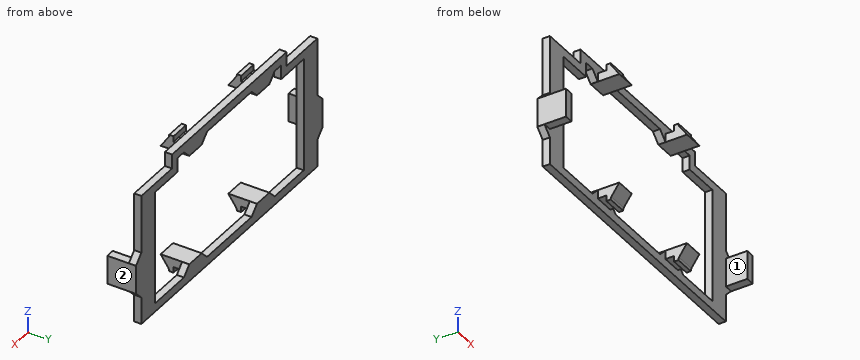
from build123d import *

# Parameters (mm, degrees)
PAD_DEPTH         = 1
SKETCH001_W       = 2.75
SKETCH001_H       = 1.2
PAD001_DEPTH      = 3
PAD001_DEPTH_BACK = 1
CHAMFER_SIZE      = 1.19
SKETCH002_W       = 2.75
SKETCH002_H       = 2
PAD002_DEPTH      = 0.6
FILLET_R          = 0.79
CHAMFER001_SIZE   = 1.19
SKETCH003_W       = 1.2
SKETCH003_H       = 4
PAD003_DEPTH      = 3
PAD003_DEPTH_BACK = 1
CHAMFER002_SIZE   = 1.19


with BuildPart() as part:
    # Sketch → Pad (new body)
    with BuildSketch(Plane.XZ):
        Polygon((-19.5, -9.15), (19.5, -9.15), (19.5, 9.15), (12.7, 9.15), (12.7, 11.15), (-12.7, 11.15), (-12.7, 9.15), (-19.5, 9.15), align=None)
        Polygon((-16.5, -7.95), (16.5, -7.95), (16.5, 7.95), (11.5, 7.95), (11.5, 9.95), (-11.5, 9.95), (-11.5, 7.95), (-16.5, 7.95), align=None, mode=Mode.SUBTRACT)
    extrude(amount=-PAD_DEPTH)

    # Sketch001 → Pad001 (join, two sides)
    with BuildSketch(Plane.XZ) as pad001_sk:
        with Locations((-7.5, 9.35)):
            Rectangle(SKETCH001_W, SKETCH001_H)
        with Locations((7.5, 9.35)):
            Rectangle(SKETCH001_W, SKETCH001_H)
        with Locations((-7.5, -7.35)):
            Rectangle(SKETCH001_W, SKETCH001_H)
        with Locations((7.5, -7.35)):
            Rectangle(SKETCH001_W, SKETCH001_H)
    extrude(amount=PAD001_DEPTH)
    extrude(pad001_sk.sketch, amount=-PAD001_DEPTH_BACK)

    # Chamfer
    chamfer_edges = [part.edges().sort_by_distance(p)[0] for p in [
        (-6.125, 0.5, -7.95),
        (-8.875, 0.5, -7.95),
        (6.125, 0.5, -7.95),
        (8.875, 0.5, -7.95),
        (8.875, 0.5, 9.95),
        (6.125, 0.5, 9.95),
        (-6.125, 0.5, 9.95),
        (-8.875, 0.5, 9.95),
    ]]
    chamfer(chamfer_edges, length=CHAMFER_SIZE)

    # Sketch002 (on DatumPlane) → Pad002 (join)
    with BuildSketch(Plane.XZ.offset(1.2)):
        with Locations((-7.5, 9.75)):
            Rectangle(SKETCH002_W, SKETCH002_H)
        with Locations((7.5, 9.75)):
            Rectangle(SKETCH002_W, SKETCH002_H)
        with Locations((7.5, -7.75)):
            Rectangle(SKETCH002_W, SKETCH002_H)
        with Locations((-7.5, -7.75)):
            Rectangle(SKETCH002_W, SKETCH002_H)
    extrude(amount=PAD002_DEPTH)

    # Fillet
    fillet_edges = [part.edges().sort_by_distance(p)[0] for p in [
        (7.5, -1.8, 9.95),
        (-7.5, -1.8, 9.95),
        (-7.5, -1.8, -7.95),
        (7.5, -1.8, -7.95),
    ]]
    fillet(fillet_edges, radius=FILLET_R)

    # Chamfer001
    chamfer001_edges = [part.edges().sort_by_distance(p)[0] for p in [
        (7.5, -3, 9.95),
        (-7.5, -3, 9.95),
        (-7.5, -3, -7.95),
        (7.5, -3, -7.95),
    ]]
    chamfer(chamfer001_edges, length=CHAMFER001_SIZE)

    # Sketch003 → Pad003 (join, two sides)
    with BuildSketch(Plane.XZ) as pad003_sk:
        with Locations((20.1, -2.15)):
            Rectangle(SKETCH003_W, SKETCH003_H)
        with Locations((-20.1, -2.15)):
            Rectangle(SKETCH003_W, SKETCH003_H)
    extrude(amount=PAD003_DEPTH)
    extrude(pad003_sk.sketch, amount=-PAD003_DEPTH_BACK)

    # Chamfer002
    chamfer002_edges = [part.edges().sort_by_distance(p)[0] for p in [
        (-19.5, 0.5, -4.15),
        (-19.5, 0.5, -0.15),
        (19.5, 0.5, -4.15),
        (19.5, 0.5, -0.15),
    ]]
    chamfer(chamfer002_edges, length=CHAMFER002_SIZE)


solid = part.part
Can you work these out from the model? Positions are in its coordinate system, mm. Face numbers are marked on the shaded views. A direction names the side the tool comes from. Coordinates: 2 decimals unless noted, no trailing zeros. Write each loop counter-clockwise with the first axis right and the second up, starting at its lowest first coordinate (ties: lowest second). Pieces come first, ordered by that corner, then holes. Notation, with made-up numbers: (62, 26.25) - (81, 26.25) arc R17 cw to (81, 58.25) - close; hole circle Ø6 at (18, -22.75). An arc over 180 degrees is marked (long way). Return JSON: item names as keys, results as strings. Group by question number.
Item 1: Which directions (+Z, -Z, +X, -X, +Y, -Y) give clear straight access to the entire face, cutting with the end or side of a thin tool? Please do the marked faces 1 and 2.
Item 2: If we section it at A-A (z = 1.5): Write out the boundary of the cut face in (x, y).
Item 3: Please list where these lines run through material, in increasing order: probe 1 along X at (y, z) = (0.3, 8); probe 2 along X at (y, z) = (-0.25, -2.75); probe 3 along Z at (x, y) = (13.5, 0.2).
Item 4: If we section it at B-B (x = -12): Write out the boundary of the cut face in (y, z), then the cut area to 3 significant figures.
Item 5: If we section it at C-C (y = -0.45): Write out the boundary of the cut face in (x, z) (3 decimals), then the cut area to 3 significant figures.
Item 6: I'm going to push flat-ended pins straight in: pin 1 Ø0.5 at (x, y) = (17, 0.5) entering from +Z; pin 2 Ø2 at (y, z) = (-2, -7.5) entering from -X (3 decimals); pin 3 Ø0.8 at (y, z) = (0.5, 8.5) entering from -X. Where does each tip first touch, or does it pass through?
Item 7: If we section it at D-D (x = -18): Write out the boundary of the cut face in (y, z).
Return value:
{
 "1": {"face 1": "+Z, -Z, -Y", "face 2": "+Z, -Z, +X, +Y, -Y"},
 "2": {"outline": "(-19.5, 0) - (-16.5, 0) - (-16.5, 1) - (-19.5, 1) - close; (16.5, 0) - (19.5, 0) - (19.5, 1) - (16.5, 1) - close"},
 "3": {"probe 1": "x = -19.5 to -11.5, 11.5 to 19.5", "probe 2": "x = -20.7 to -19.5, 19.5 to 20.7", "probe 3": "z = -9.15 to -7.95, 7.95 to 9.15"},
 "4": {"outline": "(0, -9.15) - (1, -9.15) - (1, -7.95) - (0, -7.95) - close; (0, 7.95) - (1, 7.95) - (1, 11.15) - (0, 11.15) - close", "area": "4.40 mm^2"},
 "5": {"outline": "(-20.7, -4.15) - (-19.5, -4.15) - (-19.5, -0.15) - (-20.7, -0.15) - close; (-8.875, -7.95) - (-6.125, -7.95) - (-6.125, -6.75) - (-8.875, -6.75) - close; (-8.875, 8.75) - (-6.125, 8.75) - (-6.125, 9.95) - (-8.875, 9.95) - close; (6.125, -7.95) - (8.875, -7.95) - (8.875, -6.75) - (6.125, -6.75) - close; (6.125, 8.75) - (8.875, 8.75) - (8.875, 9.95) - (6.125, 9.95) - close; (19.5, -4.15) - (20.7, -4.15) - (20.7, -0.15) - (19.5, -0.15) - close", "area": "22.8 mm^2"},
 "6": {"pin 1": "stops at z = 9.15", "pin 2": "stops at x = -8.875", "pin 3": "stops at x = -19.5"},
 "7": {"outline": "(0, -9.15) - (1, -9.15) - (1, 9.15) - (0, 9.15) - close"}
}
